```python
from build123d import *

# Parameters (mm, degrees)
SKETCH_1_W                  = 42
SKETCH_1_H                  = 42
EXTRUDE_1_DEPTH             = 2
SKETCH_2_R                  = 1
CUT_EXTRUDE_2_DEPTH         = 33.61880943
PATTERN_LINEAR_1_COUNT      = 2
PATTERN_LINEAR_1_PITCH      = 28
PATTERN_LINEAR_1_COUNT_DIR2 = 2
PATTERN_LINEAR_1_PITCH_DIR2 = 28
EXTRUDE_START               = -2
SKETCH_4_W                  = 50
SKETCH_4_H                  = 2
EXTRUDE_2_DEPTH             = 22
SKETCH_7_W                  = 40
SKETCH_7_H                  = 2
CUT_EXTRUDE_3_DEPTH         = 20
PATTERN_LINEAR_2_COUNT      = 2
PATTERN_LINEAR_2_PITCH      = 10
SKETCH_8_R                  = 1.5
CUT_EXTRUDE_4_DEPTH         = 44.995814029
PATTERN_LINEAR_3_COUNT      = 4
PATTERN_LINEAR_3_PITCH      = 5
PATTERN_LINEAR_3_COUNT_DIR2 = 2
PATTERN_LINEAR_3_PITCH_DIR2 = 45


with BuildPart() as part:
    # 草图1 → 凸台-拉伸1 (new body)
    with BuildSketch(Plane.XY):
        with Locations((-0.838569079, -3.146710526)):
            Rectangle(SKETCH_1_W, SKETCH_1_H)
    extrude(amount=EXTRUDE_1_DEPTH)

    # 草图2 → 切除-拉伸2 (cut, through all)
    with BuildSketch(Plane.XY.offset(2)):
        with Locations((-14.838569079, 10.853289474)):
            Circle(SKETCH_2_R)
    cut_extrude_2 = extrude(amount=-CUT_EXTRUDE_2_DEPTH, mode=Mode.SUBTRACT)

    # 阵列(线性)1: Cut-Extrude 2 2 × 2
    with Locations(*[(j * PATTERN_LINEAR_1_PITCH_DIR2, -i * PATTERN_LINEAR_1_PITCH, 0) for i in range(PATTERN_LINEAR_1_COUNT) for j in range(PATTERN_LINEAR_1_COUNT_DIR2) if (i, j) != (0, 0)]):
        add(cut_extrude_2, mode=Mode.SUBTRACT)

    # 草图4 → 凸台-拉伸2 (add)
    with BuildSketch(Plane.XY.offset(2).offset(EXTRUDE_START)):
        with Locations((-0.838569079, 2.853289474)):
            Rectangle(SKETCH_4_W, SKETCH_4_H)
    extrude_2 = extrude(amount=EXTRUDE_2_DEPTH)

    # 草图7 → 切除-拉伸3 (cut)
    with BuildSketch(Plane.XY.offset(22)):
        with Locations((-0.838569079, 2.853289474)):
            Rectangle(SKETCH_7_W, SKETCH_7_H)
    cut_extrude_3 = extrude(amount=-CUT_EXTRUDE_3_DEPTH, mode=Mode.SUBTRACT)

    # 阵列(线性)2: 凸台-拉伸2, 切除-拉伸3 ×2
    with Locations(*[(0, -i * PATTERN_LINEAR_2_PITCH, 0) for i in range(1, PATTERN_LINEAR_2_COUNT)]):
        add(extrude_2)
        add(cut_extrude_3, mode=Mode.SUBTRACT)

    # 草图8 → 切除-拉伸4 (cut, through all)
    with BuildSketch(Plane(origin=(0, 3.853289474, 0), x_dir=(1, 0, 0), z_dir=(0, 1, 0))):
        with Locations(Location((-23.338569079, -19, 0), (0, 0, 270))):
            Circle(SKETCH_8_R)
    cut_extrude_4 = extrude(amount=-CUT_EXTRUDE_4_DEPTH, mode=Mode.SUBTRACT)

    # 阵列(线性)3: Cut-Extrude 4 4 × 2
    with Locations(*[(j * PATTERN_LINEAR_3_PITCH_DIR2, 0, i * PATTERN_LINEAR_3_PITCH) for i in range(PATTERN_LINEAR_3_COUNT) for j in range(PATTERN_LINEAR_3_COUNT_DIR2) if (i, j) != (0, 0)]):
        add(cut_extrude_4, mode=Mode.SUBTRACT)


solid = part.part
```
Check sheet for the modelled part. Datum: model origin and axes. Units: mm. A direction names the side the tool comes from. Give positions to 0.01 mm unless a question says otherwise; leave off trailing zeros. Order: outer loops, then holes, each group sorted by start corner. A loop starts at its lowest first (then second) coordinate and runs counter-clockwise, first axis right, second up. Notation, with made-up numbers: (75.25, 40) -> (122.25, 40) arc R27 cw to (122.25, 67) -> close; hole circle Ø8 at (-27.75, -9). An arc over 180 degrees is marked (long way). Use CSV: the item, a comma, the result in double quotes. Start each with the question number.
1) Sectioned sample at A-A, the plane z = 19. Give the number of separate pieces and of enclosed holes in the cut face, plus the area to 3 significant figures.
2) Sectioned sample at C-C, the plane z = 16.25. Record the boundary of the cut face in (x, y).
3) Set-up check for faces 1 (the face through (20.161, -2, 1)), 2 (the face through (-1, 17.853, 1)): record each of +Z, -Z, +X, -X, +Y, -Y from which the full face is reachable in a straight line by a thin tool's end or side.
4) Mould release check, pull along X, two halves, no side actions. Record for faces 3 (the face through (20.161, -16, 1)), 4 (the face through (-23, 3, 22)), 5 (the face through (-15.6, 11.5, 1)), 6 (the face through (-22.325, -7.133, 17.894)): released by +X, released by -X, zero draft, split by the parting line, or undercut.
5) Go/stop test with flat-tipped pins: P1, Ø2, axis at y = -15.5, z = 1.5, coming from the -X side; P2, Ø5.5, axis at x = 21, z = 9.5, coming from the +Y side; P3, Ø8, axis at y = 8.5, z = 18.5, coming from the -X side; P4, Ø3.5, axis at x = -23.34, z = 19, coming from the -Y side. Record where each tip stops, or that it passes through.
6) Sectioned sample at D-D, the plane y = 3. Record the boundary of the cut face in (x, z), plus the area to 3 significant figures.
7) Sectioned sample at B-B, the plane x = 21. Record the boundary of the cut face in (y, z).
8) Material ranges on line 1 (X direction, y = -7, z = 19); line 2 (Y direction, x = -22, z = 16.75); line 3 (Z direction, x = -17, y = -12), recorded low to high. Write a range as from..to.
Recorded:
1,separate pieces,"8"
1,enclosed holes,"0"
1,area,"16.0 mm2"
2,outline,"(-25.84, -8.15) -> (-20.84, -8.15) -> (-20.84, -6.15) -> (-25.84, -6.15) -> close; (-25.84, 1.85) -> (-20.84, 1.85) -> (-20.84, 3.85) -> (-25.84, 3.85) -> close; (19.16, -8.15) -> (24.16, -8.15) -> (24.16, -6.15) -> (19.16, -6.15) -> close; (19.16, 1.85) -> (24.16, 1.85) -> (24.16, 3.85) -> (19.16, 3.85) -> close"
3,face 1,"+Z, -Z, +X"
3,face 2,"+Z, -Z, +X, -X, +Y"
4,face 3,"released by +X"
4,face 4,"zero draft"
4,face 5,"undercut"
4,face 6,"undercut"
5,P1,"x = -21.84"
5,P2,"y = 3.85"
5,P3,"through"
5,P4,"y = -8.15"
6,outline,"(-25.84, 0) -> (24.16, 0) -> (24.16, 22) -> (19.16, 22) -> (19.16, 2) -> (-20.84, 2) -> (-20.84, 22) -> (-25.84, 22) -> close; hole circle Ø3 at (-23.34, 19); hole circle Ø3 at (21.66, 19)"
6,area,"286 mm2"
7,outline,"(-8.15, 0) -> (-6.15, 0) -> (-6.15, 17.65) -> (-8.15, 17.65) -> close; (-8.15, 20.35) -> (-6.15, 20.35) -> (-6.15, 22) -> (-8.15, 22) -> close; (1.85, 0) -> (3.85, 0) -> (3.85, 17.65) -> (1.85, 17.65) -> close; (1.85, 20.35) -> (3.85, 20.35) -> (3.85, 22) -> (1.85, 22) -> close"
8,line 1,"-25.84..-24.84, -21.84..-20.84, 19.16..20.16, 23.16..24.16"
8,line 2,"-8.15..-6.15, 1.85..3.85"
8,line 3,"0..2"
